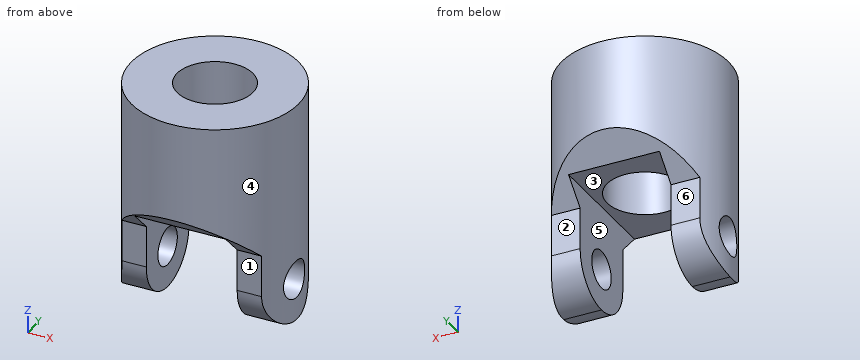
```python
from build123d import *
from OCP.BRepAlgoAPI import BRepAlgoAPI_Cut
from OCP.TopTools import TopTools_ListOfShape

# Parameters (mm, degrees)
SKETCH_1_R               = 11
EXTRUDE_1_DEPTH          = 29
CUT_EXTRUDE_1_DEPTH      = 29
CUT_EXTRUDE_1_DEPTH_BACK = 29
SKETCH_3_W               = 12
SKETCH_3_H               = 23.957820674
CUT_EXTRUDE_2_DEPTH      = 14
FILLET_START             = -11
FILLET_1_DEPTH           = 21.999997277
SKETCH_4_R               = 5
CUT_EXTRUDE_3_DEPTH      = 17
CUT_EXTRUDE_4_DEPTH      = 17
CUT_EXTRUDE_4_DEPTH_BACK = 17
SKETCH_5_R               = 2.5


with BuildPart() as part:
    # 草图1 → 凸台-拉伸1 (new body)
    with BuildSketch(Plane.XY):
        with Locations(Location((0, 0, 0), (0, 0, 180))):
            Circle(SKETCH_1_R)
    extrude(amount=EXTRUDE_1_DEPTH)

    # 草图2 → 切除-拉伸1 (cut, two sides: drawn at the far end of the back side and taken through both)
    with BuildSketch(Plane(origin=(0, 0, 0), x_dir=(0, 0, -1), z_dir=(1, 0, 0)).offset(-CUT_EXTRUDE_1_DEPTH_BACK)):
        Polygon((0, 5), (0, 11), (-17, 11), (-11, 5), align=None)
        Polygon((-17, -12), (0, -12), (0, -6), (-11, -6), align=None)
    extrude(amount=CUT_EXTRUDE_1_DEPTH + CUT_EXTRUDE_1_DEPTH_BACK, mode=Mode.SUBTRACT)

    # 草图3 → 切除-拉伸2 (cut)
    with BuildSketch(Plane(origin=(0, 0, 0), x_dir=(-1, 0, 0), z_dir=(0, 0, -1))):
        Rectangle(SKETCH_3_W, SKETCH_3_H)
    extrude(amount=-CUT_EXTRUDE_2_DEPTH, mode=Mode.SUBTRACT)


with BuildPart() as fillet_1_tool:
    # 圆角1: read off the stored shape, not the designer's step
    # 圆角1 outline → 圆角1 (new body)
    with BuildSketch(Plane.YZ.offset(FILLET_START)):
        with BuildLine():
            Line((-6, 0), (-0.5, 0))
            ThreePointArc((-0.5, 0), (-4.389087297, 1.610912703), (-6, 5.5))
            Line((-6, 5.5), (-6, 0))
        make_face()
        with BuildLine():
            ThreePointArc((5, 5.5), (3.389087297, 1.610912703), (-0.5, 0))
            Line((-0.5, 0), (5, 0))
            Line((5, 0), (5, 5.5))
        make_face()
    extrude(amount=FILLET_1_DEPTH)


with BuildPart() as part_1:
    add(part.part)

    # 圆角1: cut by fillet_1_tool, with a tolerance
    fillet_1_stock = TopTools_ListOfShape()
    fillet_1_stock.Append(part_1.part.wrapped)
    fillet_1_tools = TopTools_ListOfShape()
    fillet_1_tools.Append(fillet_1_tool.part.wrapped)
    fillet_1_cut = BRepAlgoAPI_Cut()
    fillet_1_cut.SetArguments(fillet_1_stock)
    fillet_1_cut.SetTools(fillet_1_tools)
    fillet_1_cut.SetFuzzyValue(0.00001)
    fillet_1_cut.Build()
    add(Compound.cast(fillet_1_cut.Shape()).solids(), mode=Mode.REPLACE)

    # 草图4 → 切除-拉伸3 (cut)
    with BuildSketch(Plane.XY.offset(29)):
        Circle(SKETCH_4_R)
    extrude(amount=-CUT_EXTRUDE_3_DEPTH, mode=Mode.SUBTRACT)

    # 草图5 → 切除-拉伸4 (cut, two sides: drawn at the far end of the back side and taken through both)
    with BuildSketch(Plane(origin=(-6, 0, 0), x_dir=(0, 0, -1), z_dir=(1, 0, 0)).offset(-CUT_EXTRUDE_4_DEPTH_BACK)):
        with Locations(Location((-5.5, -0.5, 0), (0, 0, 11.536959033))):
            Circle(SKETCH_5_R)
    extrude(amount=CUT_EXTRUDE_4_DEPTH + CUT_EXTRUDE_4_DEPTH_BACK, mode=Mode.SUBTRACT)


solid = part_1.part
```
Part model, mm, in its own coordinate system. Face numbers are marked on the shaded views. A direction names the side the tool comes from. Give positions to 0.01 mm unless a question says otherwise; leave off trailing zeros. Write each loop counter-clockwise with the first axis right and the second up, starting at its lowest first coordinate (ties: lowest second). Pieces come first, ordered by that corner, then holes. Notation, with made-up numbers: (61, -29.5) -> (105, -29.5) arc R13 ccw to (105, -10.5) -> close; hole circle Ø11 at (53.5, 25.5). An arc over 180 degrees is marked (long way). Put each result on its own line as item: value. Start each with the question number.
Item 1: Cut at D-D (z = 25). List the corners of the cut face in (x, y), then the cut area to 3 significant figures.
Item 2: Cut at B-B (y = 3.5). List the corners of the cut face in (x, z).
Item 3: Wall check: L1, parallel to Z at x = -7.6, y = -0.5; L2, parallel to Y at x = 0, z = 23.75; L3, parallel to Y at x = -8.15, z = 5.5. Give the ranges that are in metal, low to high. Write a range as [from, to].
Item 4: Pull direction X, two halves, no side cores. Call the marked faces 4, 5 and 6: pulls with the +X half, pulls with the -X half, needs draft (parallel to the pull), parting line crosses it, or undercut.
Item 5: Pin check, flat tips, straight feed: pin 1 Ø4 at (x, z) = (8.5, 8.5) entering from +Y; pin 2 Ø11.5 at (x, y) = (0, 0) entering from -Z; pin 3 Ø1 at (x, z) = (-7, 9) entering from -Y. Stop position of each tip, or through.
Item 6: Cut at A-A (x = 0). List the corners of the cut face in (y, z), then the cut area to 4 significant figures.
Item 7: Cut at C-C (x = 8.5). List the corners of the cut face in (y, z), then the cut area to 3 significant figures.
Item 8: Which spindle directions (+Z, -Z, +X, -X, +Y, -Y) get a long thin tool onto all of the face, cutting with end or side? Do the marked faces 1, 2 and 3. Say none if no direction does.
Answer list:
1. outline: circle Ø22 at (0, 0); hole circle Ø10 at (0, 0)
1. area: 302 mm2
2. outline: (-10.43, 1.73) -> (-6, 1.73) -> (-6, 14) -> (-3.57, 14) -> (-3.57, 29) -> (-10.43, 29) -> close; (3.57, 14) -> (6, 14) -> (6, 1.73) -> (10.43, 1.73) -> (10.43, 29) -> (3.57, 29) -> close
3. L1: z = [0, 3], [8, 29]
3. L2: y = [-11, -5], [5, 11]
3. L3: y = [-6, -3], [2, 5]
4. face 4: parting line crosses it
4. face 5: undercut
4. face 6: needs draft
5. pin 1: stops at y = 5
5. pin 2: stops at z = 14
5. pin 3: stops at y = -6
6. outline: (-11, 16) -> (-9, 14) -> (-5, 14) -> (-5, 29) -> (-11, 29) -> close; (5, 14) -> (8, 14) -> (11, 17) -> (11, 29) -> (5, 29) -> close
6. area: 173.5 mm2
7. outline: (-6.98, 11.98) -> (-6, 11) -> (-6, 5.5) arc R5.5 ccw to (5, 5.5) -> (5, 11) -> (6.98, 12.98) -> (6.98, 29) -> (-6.98, 29) -> close; hole circle Ø5 at (-0.5, 5.5)
7. area: 337 mm2
8. face 1: -Z, +X, -X, -Y
8. face 2: -Z, +X, -X, +Y
8. face 3: -Z, +Y, -Y
